Autodesk Inventor part; units mm, degrees
ref_plane "YZ Plane" through (0, 0, 0) normal (1, 0, 0) x (0, 1, 0)
ref_plane "XZ Plane" through (0, 0, 0) normal (0, 1, 0) x (-1, 0, 0)
ref_plane "XY Plane" through (0, 0, 0) normal (0, 0, 1) x (1, 0, 0)
sketch "Sketch1" plane through (0, 0, 0) normal (0, 0, 1) x (1, 0, 0)
  circle A0 centre (0, 0) radius 2.3114
  circle A1 centre (25.4, 0) radius 2.3114
  circle A2 centre (50.8, 0) radius 2.3114
  arc A3 (0, 6.35) -> (0, -6.35) centre (0, 0) ccw
  arc A4 (50.8, -6.35) -> (50.8, 6.35) centre (50.8, 0) ccw
  line L0 (0, 6.35) -> (50.8, 6.35)
  line L1 (0, -6.35) -> (50.8, -6.35)
  dimension "d0" = 4.6228
  dimension "d1" = 4.6228
  dimension "d2" = 4.6228
  dimension "d3" = 12.7
  dimension "d5" = 12.7
extrude "Extrusion1" add sketch "Sketch1" along normal blind 1.5875
properties part number "Joint Gusset" material "Acetal Resin, White"
Can you work these out from the model? Positions are in its coordinate system, mm. Give positions to 0.01 mm unless a question says otherwise; leave off trailing zeros. Order: outer loops, then holes, each group sorted by start corner. A loop starts at its lowest first (then second) coordinate and runs counter-clockwise, first axis right, second up. Notation, with made-up numbers: M 10,57 L 40,57 A18 ccw 40,83 Z; hole C -31.5,66.25 d1. An arc over 180 degrees is marked long. Use a Markdown table: item, result. Add a question column.
Item 1: Suppose I cut it at C-C (z = 0.95). List the corners of the cut face in (x, y) for me.
Item 2: Suppose I cut it at B-B (y = 0). List the corners of the cut face in (x, z) for me, then the cut area to 3 significant figures.
Item 3: If I drill on L1, parallel to Y at x = 50.8, z = 0.9; L2, parallel to X at y = -2, z = 0.35, over which ranges is the centre line in solid material (lowest first)? Write a range as [from, to].
Item 4: Suppose I cut it at D-D (x = 51.5). List the corners of the cut face in (y, z) for me.
Item 5: Suppose I cut it at A-A (x = 25.4). List the corners of the cut face in (y, z) for me, then the cut area to 3 significant figures.
Item 6: We'd pull the mould along X, two halves only. Please class faces 1 (the cylindrical face through (23.09, -0.1, 0.78)), 2 (the flat face through (25, 6.35, 1)), 3 (the cylindrical face through (57.15, 0.14, 0.78)): +X half, -X half, draft (parallel to the pull), parting line (faces both ways), or undercut.
Answer sheet:
| question | item | result |
|---|---|---|
| 1 | outline | M 0,-6.35 L 50.8,-6.35 A6.35 ccw 50.8,6.35 L 0,6.35 A6.35 ccw Z; hole C 0,0 d4.62; hole C 25.4,0 d4.62; hole C 50.8,0 d4.62 |
| 2 | outline | M -6.35,0 L -2.31,0 L -2.31,1.59 L -6.35,1.59 Z; M 2.31,0 L 23.09,0 L 23.09,1.59 L 2.31,1.59 Z; M 27.71,0 L 48.49,0 L 48.49,1.59 L 27.71,1.59 Z; M 53.11,0 L 57.15,0 L 57.15,1.59 L 53.11,1.59 Z |
| 2 | area | 78.8 mm² |
| 3 | L1 | y = [-6.35, -2.31], [2.31, 6.35] |
| 3 | L2 | x = [-6.03, -1.16], [1.16, 24.24], [26.56, 49.64], [51.96, 56.83] |
| 4 | outline | M -6.31,0 L -2.2,0 L -2.2,1.59 L -6.31,1.59 Z; M 2.2,0 L 6.31,0 L 6.31,1.59 L 2.2,1.59 Z |
| 5 | outline | M -6.35,0 L -2.31,0 L -2.31,1.59 L -6.35,1.59 Z; M 2.31,0 L 6.35,0 L 6.35,1.59 L 2.31,1.59 Z |
| 5 | area | 12.8 mm² |
| 6 | face 1 | undercut |
| 6 | face 2 | draft |
| 6 | face 3 | +X half |
